Print and shaded views of the part. All mm, measured from the part's lowest x, y and z. A direction names the side the tool comes from. Coordinates: 2 decimals unless noted, no trailing zeros. Loops run counter-clockwise (first coordinate to the right, second up) from the corner with the lowest first, then second, coordinate; pieces in that order, holes last.
1) Saw through at C-C, the plane z = 3. Write the cut outline in (x, y).
2) Pin check, flat tip, straight feed: pin 1 Ø4.5 at (x, z) = (7.5, 24) entering from -Y. Stop position of the tip, or through.
3) Which spindle directions (+Z, -Z, +X, -X, +Y, -Y) get a long thin tool onto all of the face, cutting with end or side? Do the marked faces 5 and 6. Say none if no direction does.
4) Saw through at A-A, the plane x = 7.5. Give the number of separate pieces and of enclosed holes in the cut face, and give its area (3 significant figures).
5) Wall check: line 1 along Z through (x, y) = (1.75, 11); line 2 along Y through (x, z) = (10.75, 11.5); line 3 along X through (y, z) = (6.5, 20). Give the ranges that are in metal, low to high.
6) Saw through at D-D, the plane z = 40. Write the cut outline in (x, y).
7) Two-plate mould, pull along Y, no slides. Class the marked faces 1, 2, 3 and 4: +Y half, -Y half, draft (parallel to the pull), parting line (faces both ways), or undercut.
8) Saw through at B-B, the plane y = 8.75. Write the cut outline in (x, z).
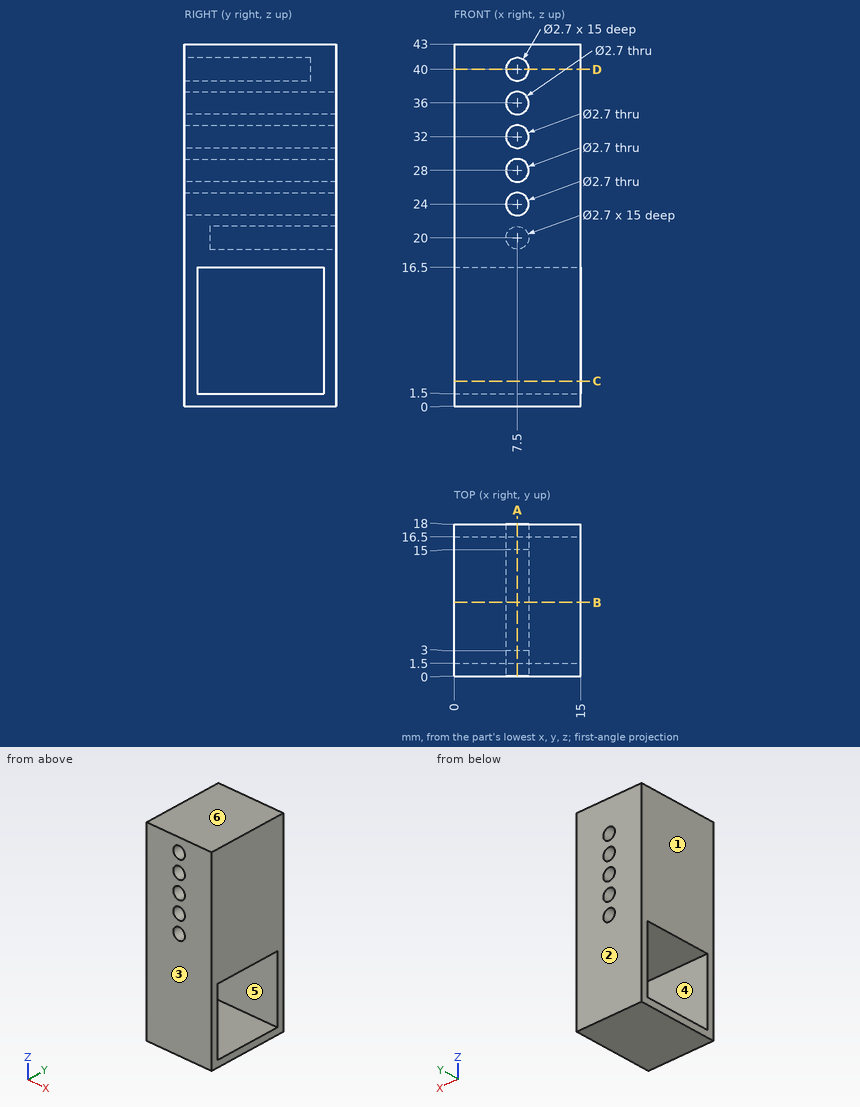
Data:
1. outline: (0, 0) - (15, 0) - (15, 1.5) - (0, 1.5) - close; (0, 16.5) - (15, 16.5) - (15, 18) - (0, 18) - close
2. pin 1: stops at y = 0
3. face 5: +X, -X
3. face 6: +Z, +X, -X, +Y, -Y
4. separate pieces: 5
4. enclosed holes: 1
4. area: 274 mm2
5. line 1: z = 0 to 1.5, 16.5 to 43
5. line 2: y = 0 to 1.5, 16.5 to 18
5. line 3: x = 0 to 6.15, 8.85 to 15
6. outline: (0, 0) - (6.15, 0) - (6.15, 15) - (8.85, 15) - (8.85, 0) - (15, 0) - (15, 18) - (0, 18) - close
7. face 1: draft
7. face 2: +Y half
7. face 3: -Y half
7. face 4: undercut
8. outline: (0, 0) - (15, 0) - (15, 1.5) - (0, 1.5) - close; (0, 16.5) - (15, 16.5) - (15, 43) - (0, 43) - close; hole circle Ø2.7 at (7.5, 20); hole circle Ø2.7 at (7.5, 24); hole circle Ø2.7 at (7.5, 28); hole circle Ø2.7 at (7.5, 32); hole circle Ø2.7 at (7.5, 36); hole circle Ø2.7 at (7.5, 40)
